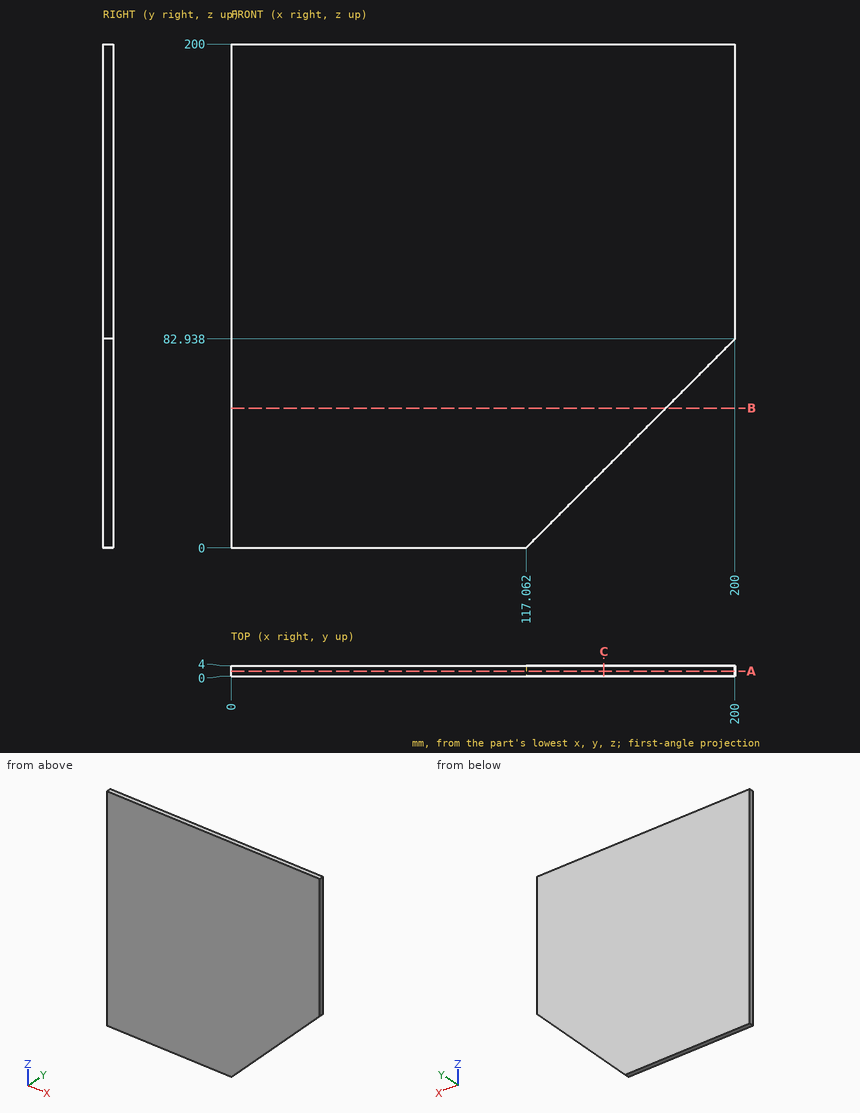
The drawing under review shows one solid part. Ordinate dimensions are in mm from its lowest x, y, z. Coordinates: 2 decimals unless noted, no trailing zeros. Write each loop counter-clockwise with the first axis right and the second up, starting at its lowest first coordinate (ties: lowest second). Pieces come first, ordered by that corner, then holes. Notation, with made-up numbers: (2.5, -24) - (23.5, -24) arc R9 cw to (23.5, -19) - close; hole circle Ø5 at (-36.75, -1). An arc over 180 degrees is marked (long way). Answer in a Markdown table with one row per item. Add a question column.
Q1. For probe 1 along Z at (x, y) = (184, 0.4); probe 2 along X at (y, z) = (2.45, 72); probe 3 along X at (y, z) = (1.1, 76), list the stretches that pass through material, from the lowest coordinate up.
Q2. For P1, Ø12, axis at x = 70, z = 30.5, coming from the -Y side, flat-tipped, find the tip position at first contact; note if it passes through.
Q3. We need section C-C, the plane x = 148. State the section outline as (y, z) points, and give its area (3 significant figures).
Q4. We need section B-B, the plane z = 55.5. State the section outline as (x, y) points, and give its area (3 significant figures).
Q5. We need section A-A, the plane y = 1.9. State the section outline as (x, z) points, and give its area (3 significant figures).
Answer list:
| question | item | result |
|---|---|---|
| 1 | probe 1 | z = 66.94 to 200 |
| 1 | probe 2 | x = 0 to 189.06 |
| 1 | probe 3 | x = 0 to 193.06 |
| 2 | P1 | stops at y = 0 |
| 3 | outline | (0, 30.94) - (4, 30.94) - (4, 200) - (0, 200) - close |
| 3 | area | 676 mm2 |
| 4 | outline | (0, 0) - (172.56, 0) - (172.56, 4) - (0, 4) - close |
| 4 | area | 690 mm2 |
| 5 | outline | (0, 0) - (117.06, 0) - (200, 82.94) - (200, 200) - (0, 200) - close |
| 5 | area | 36,600 mm2 |
